Input: dimensioned drawing with shaded views. Units: mm. Origin: part minimum x, y, z. Give positions to 0.01 mm unless a question says otherwise; leave off trailing zeros. Loops run counter-clockwise (first coordinate to the right, second up) from the corner with the lowest first, then second, coordinate; pieces in that order, holes last. Notation, with made-up numbers: M -5.5,15.5 L 22.5,15.5 A25 ccw 22.5,49.5 Z; hole C 12,49.25 d6. An arc over 180 degrees is marked long. Answer in a Markdown table with one row per item.
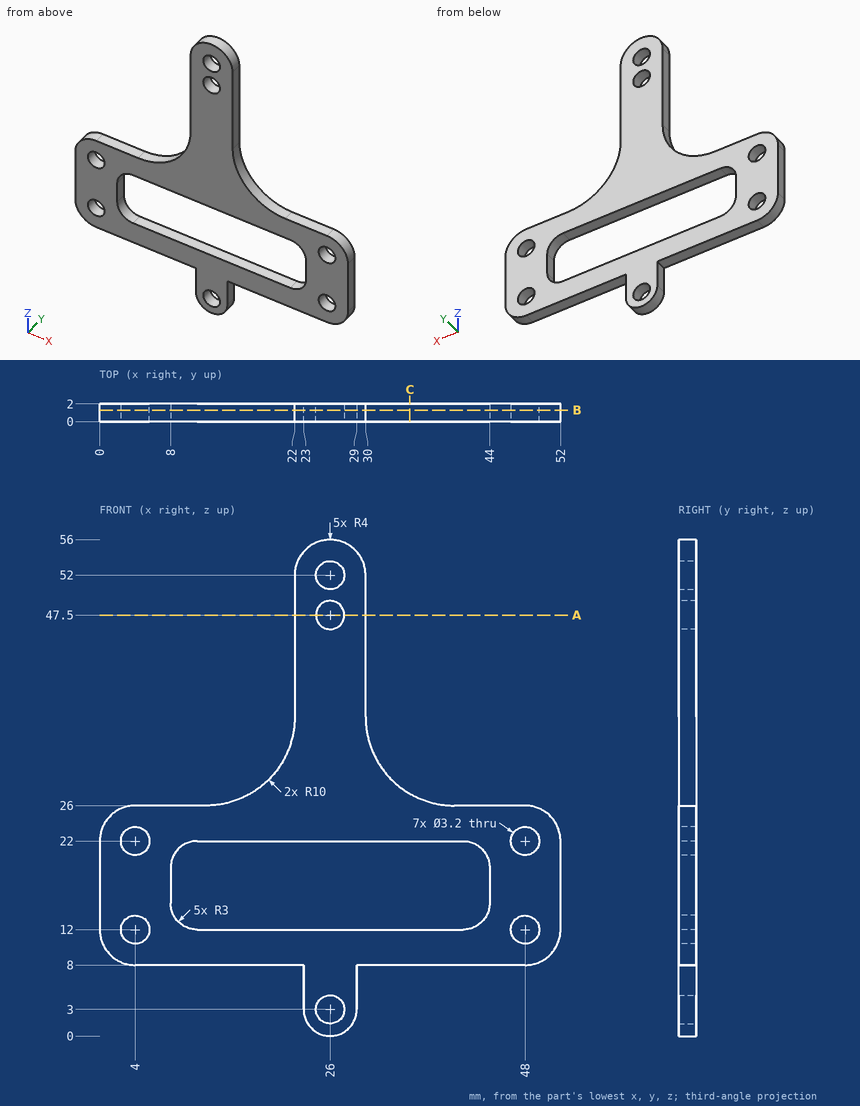
Q1. Section query B-B (y = 1.3). Give the number of separate pieces and of enclosed holes in the cut face, plus the area to 3 significant figures.
Values follow:
| item | result |
|---|---|
| separate pieces | 1 |
| enclosed holes | 8 |
| area | 834 mm^2 |
Q2. Ray query, probe 1 along Z at (x, y) = (48, 0.9); probe 2 along Z at (x, y) = (26, 1.2); probe 3 along Z at (x, y) = (20, 0.5). Return the intervals inside material, ascending. Write a range as from..to.
Values follow:
| item | result |
|---|---|
| probe 1 | 8..10.4, 13.6..20.4, 23.6..26 |
| probe 2 | 0..1.4, 4.6..12, 22..45.9, 49.1..50.4, 53.6..56 |
| probe 3 | 8..12, 22..30 |
Q3. Section query C-C (x = 35). Output: boundary loops of the cut face in (y, z), plus the area to 3 significant figures.
Values follow:
| item | result |
|---|---|
| outline | M 0,8 L 2,8 L 2,12 L 0,12 Z; M 0,22 L 2,22 L 2,27.34 L 0,27.34 Z |
| area | 18.7 mm^2 |
Q4. Contact query for flat-ended pins moving along their axis: pin 1 Ø0.6 at (y, z) = (0.5, 46.5) entering from +X; pin 2 Ø0.6 at (y, z) = (1, 42) entering from -X; pin 3 Ø3 at (x, z) = (27, 38) entering from -Y; pin 4 Ø3 at (x, z) = (4, 12) entering from -Y. Output: stop coordinate, or through.
Values follow:
| item | result |
|---|---|
| pin 1 | x = 30 |
| pin 2 | x = 22 |
| pin 3 | y = 0 |
| pin 4 | through |
Q5. Section query A-A (z = 47.5). Output: boundary loops of the cut face in (x, y), plus the area to 3 significant figures.
Values follow:
| item | result |
|---|---|
| outline | M 22,0 L 24.4,0 L 24.4,2 L 22,2 Z; M 27.6,0 L 30,0 L 30,2 L 27.6,2 Z |
| area | 9.60 mm^2 |
